Verification items for this drawing (mm, ordinates from the low corner). A direction names the side the tool comes from. Give positions to 0.01 mm unless a question says otherwise; leave off trailing zeros. Loops run counter-clockwise (first coordinate to the right, second up) from the corner with the lowest first, then second, coordinate; pieces in that order, holes last. Notation, with made-up numbers: M -26,80 L 28,80 A20 ccw 28,89 Z; hole C -40,-9.75 d4. An arc over 180 degrees is marked long. Put each result on its own line as item: value. Start each with the question number.
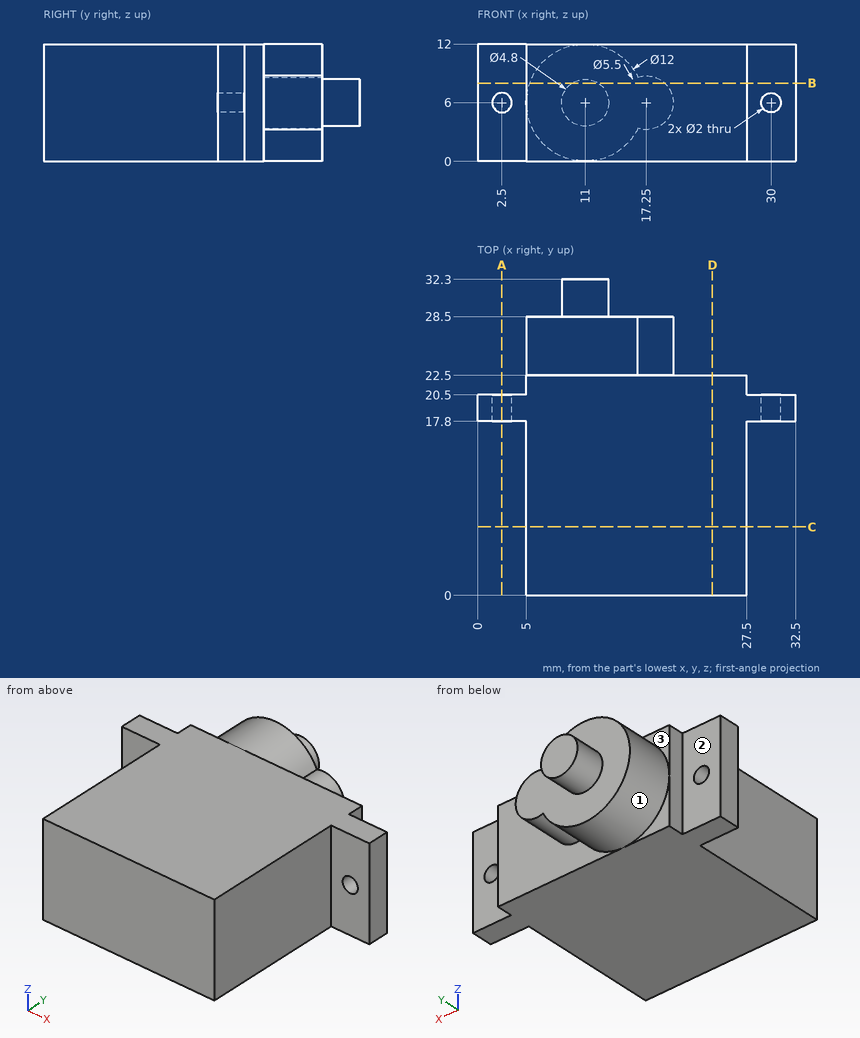
Q1. Cross-section at A-A, the plane x = 2.5. Record the boundary of the cut face in (y, z).
Q2. Scan lines: L1, parallel to X at y = 18.55, z = 6; L2, parallel to Z at x = 30, y = 19.45; L3, parallel to Y at x = 24, z = 6.75. Record each from-to range of solid material in increasing order.
Q3. Cross-section at B-B, the plane z = 8. Record the boundary of the cut face in (x, y).
Q4. Cross-section at C-C, the plane y = 7. Record the boundary of the cut face in (x, z).
Q5. Cross-section at D-D, the plane x = 24. Record the boundary of the cut face in (y, z).
Q6. Go/stop test with flat-tipped pins: pin 1 (1.8 mm diameter, centred on x = 7, z = 3.5, fed in from +Y); pin 2 (1 mm diameter, centred on y = 21.5, z = 4.5, fed in from +X); pin 3 (4 mm diameter, centred on x = 30.5, z = 6.5, fed in from -Y). Record where each tip stops, or that it passes through.
Q7. Set-up check for the marked faces 1, 2 and 3: record each of +Z, -Z, +X, -X, +Y, -Y from which the full face is reachable in a straight line by a thin tool's end or side.
Ans:
1. outline: M 17.8,0 L 20.5,0 L 20.5,5 L 17.8,5 Z; M 17.8,7 L 20.5,7 L 20.5,12 L 17.8,12 Z
2. L1: x = 0 to 1.5, 3.5 to 29, 31 to 32.5
2. L2: z = 0 to 5, 7 to 12
2. L3: y = 0 to 22.5
3. outline: M 0,17.8 L 5,17.8 L 5,0 L 27.5,0 L 27.5,17.8 L 32.5,17.8 L 32.5,20.5 L 27.5,20.5 L 27.5,22.5 L 19.14,22.5 L 19.14,28.5 L 12.33,28.5 L 12.33,32.3 L 9.67,32.3 L 9.67,28.5 L 5.34,28.5 L 5.34,22.5 L 5,22.5 L 5,20.5 L 0,20.5 Z
4. outline: M 5,0 L 27.5,0 L 27.5,12 L 5,12 Z
5. outline: M 0,0 L 22.5,0 L 22.5,12 L 0,12 Z
6. pin 1: stops at y = 28.5
6. pin 2: stops at x = 27.5
6. pin 3: stops at y = 17.8
7. face 1: +Y
7. face 2: +Z, -Z, -X, +Y
7. face 3: +Z, -X, +Y
